from build123d import *

# Parameters (mm, degrees)
SKETCH1_W              = 965.2
SKETCH1_H              = 508
BOSS_EXTRUDE1_DEPTH    = 50.8
CUT_EXTRUDE3_START     = 31.75
CUT_EXTRUDE3_OUTLINE_R = 12.7
CUT_EXTRUDE3_DEPTH     = 19.05


# Read off the part's stored shape, not the designer's step: Cut-Extrude3
with BuildPart() as part:
    # Sketch1 → Boss-Extrude1 (new body)
    with BuildSketch(Plane(origin=(0, 0, 0), x_dir=(1, 0, 0), z_dir=(0, 1, 0))):
        Rectangle(SKETCH1_W, SKETCH1_H)
    extrude(amount=BOSS_EXTRUDE1_DEPTH)

    # Cut-Extrude3 outline → Cut-Extrude3 (cut)
    with BuildSketch(Plane(origin=(0, 0, 0), x_dir=(1, 0, 0), z_dir=(0, 1, 0)).offset(CUT_EXTRUDE3_START)):
        with Locations((-254, 228.6)):
            Circle(CUT_EXTRUDE3_OUTLINE_R)
        with Locations((-254, -228.6)):
            Circle(CUT_EXTRUDE3_OUTLINE_R)
        with Locations((254, -228.6)):
            Circle(CUT_EXTRUDE3_OUTLINE_R)
        with Locations((254, 228.6)):
            Circle(CUT_EXTRUDE3_OUTLINE_R)
    extrude(amount=CUT_EXTRUDE3_DEPTH, mode=Mode.SUBTRACT)


solid = part.part
Source: CAD feature listing. Evaluate the final solid. Frame: model axes, mm. A direction names the side the tool comes from. Round coordinates to 2 decimals unless told otherwise and drop trailing zeros. Loops run counter-clockwise (first coordinate to the right, second up) from the corner with the lowest first, then second, coordinate; pieces in that order, holes last. Notation, with made-up numbers: M 26.25,47.5 L 46.25,47.5 A18 ccw 46.25,65.5 Z; hole C 48.25,4 d5. An arc over 180 degrees is marked long. Return JSON: item names as keys, results as strings. Group by question number.
1. Mould query, pull axis X, two halves, no side actions, for faces 1 (the face through (482.6, 25, 4)), 2 (the face through (254, 31.75, 228)), 3 (the face through (-7, 25, -254)). Classes: released by +X, released by -X, zero draft, split by the parting line, or undercut.
2. Section query A-A on x = 254. Output: boundary loops of the cut face in (y, z).
3. Section query B-B on z = 228.6. Output: boundary loops of the cut face in (x, y), and give its area (3 significant figures).
4. Material intervals for line 1 along X through (y, z) = (41.25, 228.6); line 2 along Z through (x, y) = (-254, 44.75), sorted ascending. Write a range as from..to.
5. Reachability of faces 4 (the face through (266.114, 41.142, 224.785)), 5 (the face through (-7, 25, 254)) from +Z, -Z, +X, -X, +Y, -Y: full face, straight path, thin tool, end or side. Return the list, or none.
6. Pin query (flat end, axial travel): pin 1 (15 mm diameter, centred on x = 254, z = 228.6, fed in from +Y); pin 2 (1.5 mm diameter, centred on x = -205.5, z = -89.5, fed in from -Y). Return the tip coordinate at first contact, or that it passes through.
Checks:
{
 "1": {"face 1": "released by +X", "face 2": "undercut", "face 3": "zero draft"},
 "2": {"outline": "M 0,-254 L 50.8,-254 L 50.8,-241.3 L 31.75,-241.3 L 31.75,-215.9 L 50.8,-215.9 L 50.8,215.9 L 31.75,215.9 L 31.75,241.3 L 50.8,241.3 L 50.8,254 L 0,254 Z"},
 "3": {"outline": "M -482.6,0 L 482.6,0 L 482.6,50.8 L 266.7,50.8 L 266.7,31.75 L 241.3,31.75 L 241.3,50.8 L -241.3,50.8 L -241.3,31.75 L -266.7,31.75 L -266.7,50.8 L -482.6,50.8 Z", "area": "48,100 mm²"},
 "4": {"line 1": "x = -482.6..-266.7, -241.3..241.3, 266.7..482.6", "line 2": "z = -254..-241.3, -215.9..215.9, 241.3..254"},
 "5": {"face 4": "+Y", "face 5": "+Z, +X, -X, +Y, -Y"},
 "6": {"pin 1": "stops at y = 31.75", "pin 2": "stops at y = 0"}
}
